CAD build for the part. Positions are in the model's coordinates, mm. A direction names the side the tool comes from. Give positions to 0.01 mm unless a question says otherwise; leave off trailing zeros. Order: outer loops, then holes, each group sorted by start corner. A loop starts at its lowest first (then second) coordinate and runs counter-clockwise, first axis right, second up.
from build123d import *

# Parameters (mm, degrees)
SKETCH1_R           = 6.35
SKETCH1_R_2         = 2.75
BOSS_EXTRUDE1_DEPTH = 12.7
SKETCH2_R           = 15.875
SKETCH2_R_2         = 2.54
SKETCH2_R_3         = 6.35
BOSS_EXTRUDE2_DEPTH = 3.175


with BuildPart() as part:
    # Sketch1 → Boss-Extrude1 (new body)
    with BuildSketch(Plane(origin=(0, 0, 0), x_dir=(1, 0, 0), z_dir=(0, 1, 0))):
        with Locations(Location((0, 0, 0), (0, 0, 270))):
            Circle(SKETCH1_R)
        with Locations(Location((0, 0, 0), (0, 0, 270))):
            Circle(SKETCH1_R_2, mode=Mode.SUBTRACT)
    extrude(amount=BOSS_EXTRUDE1_DEPTH)

    # Sketch2 → Boss-Extrude2 (add)
    with BuildSketch(Plane.XZ):
        with Locations(Location((0, 0, 0), (0, 0, 270))):
            Circle(SKETCH2_R)
        with Locations(Location((0, 11.1125, 0), (0, 0, 270))):
            Circle(SKETCH2_R_2, mode=Mode.SUBTRACT)
        with Locations(Location((0, 0, 0), (0, 0, 270))):
            Circle(SKETCH2_R_3, mode=Mode.SUBTRACT)
        with Locations(Location((11.1125, 0, 0), (0, 0, 270))):
            Circle(SKETCH2_R_2, mode=Mode.SUBTRACT)
        with Locations(Location((0, -11.1125, 0), (0, 0, 270))):
            Circle(SKETCH2_R_2, mode=Mode.SUBTRACT)
        with Locations(Location((-11.1125, 0, 0), (0, 0, 270))):
            Circle(SKETCH2_R_2, mode=Mode.SUBTRACT)
    extrude(amount=-BOSS_EXTRUDE2_DEPTH)


solid = part.part
1. Saw through at C-C on z = -10.5. Give the cut face in (x, y) (3 decimals).
2. 3-axis set-ups, long thin cutter, end or side, ignore diameter. For faces 4 (the flat face through (-7, 3.175, 0)), 5 (the cylindrical face through (-15.497, 1.565, 3.441)): which of +Z, -Z, +X, -X, +Y, -Y reach the whole face in a straight line?
3. Saw through at D-D on y = 6.25. Give the cut face in (x, z), plus the area to 3 significant figures.
4. Saw through at A-A on x = 0. State how many separate pieces and enclosed holes the cut face has, plus the area to 3 significant figures.
5. Wall check: line 1 (X direction, y = 7.5, z = 0); line 2 (Z direction, x = 1, y = 3); line 3 (Y direction, x = 10, z = 5.5) (3 decimals). Give the ranges that are in metal, low to high.
6. Pin check, flat tips, straight feed: P1, Ø8, axis at x = -11.11, z = 0, coming from the +Y side (3 decimals); P2, Ø1, axis at x = 6, y = 9.5, coming from the -Z side; P3, Ø4, axis at x = -7, y = 10, coming from the +Z side. Stop position of each tip, or through.
7. Mould opens along X. For faces 1 (the cylindrical face through (-3.86, 7.87, -5.04)), 2 (the flat face through (-1, 12.7, 3)), 3 (the cylindrical face through (-2.685, 6.261, -0.596)) say: released by +X, released by -X, zero draft, split by the parting line, or undercut.
Reported:
1. outline: (-11.907, 0) - (-2.465, 0) - (-2.465, 3.175) - (-11.907, 3.175) - close; (2.465, 0) - (11.907, 0) - (11.907, 3.175) - (2.465, 3.175) - close
2. face 4: +Y
2. face 5: +Y, -Y
3. outline: circle Ø12.7 at (0, 0); hole circle Ø5.5 at (0, 0)
3. area: 103 mm2
4. separate pieces: 4
4. enclosed holes: 0
4. area: 120 mm2
5. line 1: x = -6.35 to -2.75, 2.75 to 6.35
5. line 2: z = -15.84 to -13.45, -8.78 to -2.56, 2.56 to 8.78, 13.45 to 15.84
5. line 3: y = 0 to 3.175
6. P1: stops at y = 3.175
6. P2: stops at z = -3.17
6. P3: stops at z = 3.91
7. face 1: split by the parting line
7. face 2: zero draft
7. face 3: undercut
